```python
from build123d import *

# Parameters (mm, degrees)
SKETCH1_R           = 2.5
BOSS_EXTRUDE1_DEPTH = 105
FILLET1_R           = 0.5
FILLET2_R           = 0.5
FILLET3_R           = 1


with BuildPart() as part:
    # Sketch1 → Boss-Extrude1 (new, symmetric)
    with BuildSketch(Plane.XY):
        Polygon((3.9, -2.839339828), (6.560660172, -5.5), (8.200660172, -5.5), (8.200660172, -3.1), (9.3, -3.1), (10, -3.8), (10, -10), (3.8, -10), (3.1, -9.3), (3.1, -8.200660172), (5.5, -8.200660172), (5.5, -6.560660172), (2.839339828, -3.9), (-2.839339828, -3.9), (-5.5, -6.560660172), (-5.5, -8.200660172), (-3.1, -8.200660172), (-3.1, -9.3), (-3.8, -10), (-10, -10), (-10, -3.8), (-9.3, -3.1), (-8.200660172, -3.1), (-8.200660172, -5.5), (-6.560660172, -5.5), (-3.9, -2.839339828), (-3.9, 2.839339828), (-6.560660172, 5.5), (-8.200660172, 5.5), (-8.200660172, 3.1), (-9.3, 3.1), (-10, 3.8), (-10, 10), (-3.8, 10), (-3.1, 9.3), (-3.1, 8.200660172), (-5.5, 8.200660172), (-5.5, 6.560660172), (-2.839339828, 3.9), (2.839339828, 3.9), (5.5, 6.560660172), (5.5, 8.200660172), (3.1, 8.200660172), (3.1, 9.3), (3.8, 10), (10, 10), (10, 3.8), (9.3, 3.1), (8.200660172, 3.1), (8.200660172, 5.5), (6.560660172, 5.5), (3.9, 2.839339828), align=None)
        Circle(SKETCH1_R, mode=Mode.SUBTRACT)
    extrude(amount=BOSS_EXTRUDE1_DEPTH, both=True)

    # Fillet1
    fillet1_edges = [part.edges().sort_by_distance(p)[0] for p in [
        (-2.839339828, 3.9, 0),
        (2.839339828, 3.9, 0),
        (3.9, 2.839339828, 0),
        (3.9, -2.839339828, 0),
        (2.839339828, -3.9, 0),
        (-2.839339828, -3.9, 0),
        (-3.9, -2.839339828, 0),
        (-3.9, 2.839339828, 0),
    ]]
    fillet(fillet1_edges, radius=FILLET1_R)

    # Fillet2
    fillet2_edges = [part.edges().sort_by_distance(p)[0] for p in [
        (-5.5, 6.560660172, 0),
        (5.5, 6.560660172, 0),
        (5.5, 8.200660172, 0),
        (3.1, 8.200660172, 0),
        (8.200660172, 3.1, 0),
        (8.200660172, 5.5, 0),
        (6.560660172, 5.5, 0),
        (6.560660172, -5.5, 0),
        (8.200660172, -5.5, 0),
        (8.200660172, -3.1, 0),
        (3.1, -8.200660172, 0),
        (5.5, -8.200660172, 0),
        (5.5, -6.560660172, 0),
        (-5.5, -6.560660172, 0),
        (-5.5, -8.200660172, 0),
        (-3.1, -8.200660172, 0),
        (-8.200660172, -3.1, 0),
        (-8.200660172, -5.5, 0),
        (-6.560660172, -5.5, 0),
        (-6.560660172, 5.5, 0),
        (-8.200660172, 5.5, 0),
        (-8.200660172, 3.1, 0),
        (-3.1, 8.200660172, 0),
        (-5.5, 8.200660172, 0),
    ]]
    fillet(fillet2_edges, radius=FILLET2_R)

    # Fillet3
    fillet3_edges = [part.edges().sort_by_distance(p)[0] for p in [
        (10, 10, 0),
        (10, -10, 0),
        (-10, -10, 0),
        (-10, 10, 0),
    ]]
    fillet(fillet3_edges, radius=FILLET3_R)


solid = part.part
```
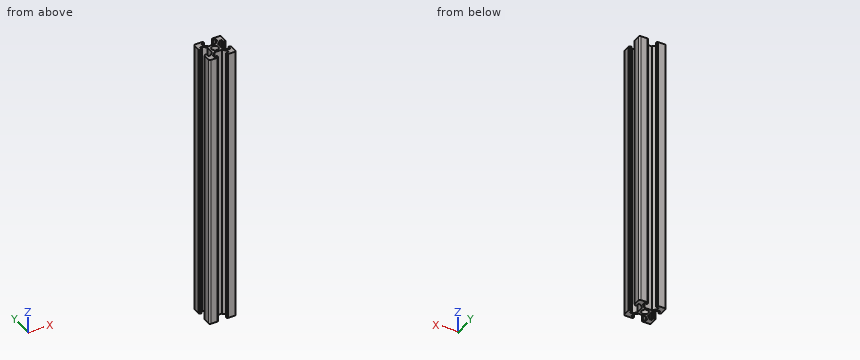
Geometry: final body of the model. Coordinates: model frame, mm. Coordinates: 2 decimals unless noted, no trailing zeros. Write each loop counter-clockwise with the first axis right and the second up, starting at its lowest first coordinate (ties: lowest second). Pieces come first, ordered by that corner, then holes. Notation, with made-up numbers: M 72,77 L 83,77 A21 ccw 83,90 Z; hole C 53.25,79.25 d6. An arc over 180 degrees is marked long. Answer as CSV lines item,"result". Start each with the question number.
Q1. Pin query (flat end, axial travel): P1, Ø1.6, axis at y = 0.5, z = 48, coming from the -X side; P2, Ø2.5, axis at y = -1, z = 29, coming from the +X side. Return the tip coordinate at first contact, or that it passes through.
Q2. Cut plane A-A on x = 0. Return the cut outline in (y, z), then the cut area to 3 significant figures.
Q3. Line query: line 1 (Y direction, x = 0, z = 41); line 2 (X direction, y = -4.25, z = 21.5); line 3 (Y direction, x = -9, z = 21.5). Output: solid intervals per line, ascending. Write a range as from..to.
Findings below:
1,P1,"stops at x = -3.9"
1,P2,"stops at x = 3.9"
2,outline,"M -3.9,-105 L -2.5,-105 L -2.5,105 L -3.9,105 Z; M 2.5,-105 L 3.9,-105 L 3.9,105 L 2.5,105 Z"
2,area,"588 mm2"
3,line 1,"y = -3.9..-2.5, 2.5..3.9"
3,line 2,"x = -10..-8.2, -5.31..-3.19, 3.19..5.31, 8.2..10"
3,line 3,"y = -10..-3.1, 3.1..10"
